```python
from build123d import *

# Parameters (mm, degrees)
SKETCH1_R           = 5
SKETCH1_R_2         = 6
SKETCH1_R_3         = 3
SKETCH1_R_4         = 4
BOSS_EXTRUDE1_DEPTH = 8


with BuildPart() as part:
    # Sketch1 → Boss-Extrude1 (new body)
    # profile 1 of 3: a face of its own
    with BuildSketch(Plane.XY):
        with BuildLine():
            Line((13.16300623, -179.16324922), (6, -179.16324922))
            ThreePointArc((6, -179.16324922), (4.585786438, -178.577462783), (4, -177.16324922))
            Line((4, -177.16324922), (4, -6.92820323))
            ThreePointArc((4, -6.92820323), (0, 8), (-4, -6.92820323))
            Line((-4, -6.92820323), (-4, -177.16324922))
            ThreePointArc((-4, -177.16324922), (-4.585786438, -178.577462783), (-6, -179.16324922))
            Line((-6, -179.16324922), (-12.83699377, -179.16324922))
            Line((-12.83699377, -179.16324922), (-12.83699377, -199.16324922))
            Line((-12.83699377, -199.16324922), (13.16300623, -199.16324922))
            Line((13.16300623, -199.16324922), (13.16300623, -179.16324922))
        make_face()
        Circle(SKETCH1_R, mode=Mode.SUBTRACT)
        with Locations((0.16300623, -189.16324922)):
            Circle(SKETCH1_R_2, mode=Mode.SUBTRACT)
        with BuildLine():
            ThreePointArc((-2, -175.16324922), (0, -177.16324922), (2, -175.16324922))
            Line((2, -175.16324922), (2, -11.176871049))
            ThreePointArc((2, -11.176871049), (0, -8.621835967), (-2, -11.176871049))
            Line((-2, -11.176871049), (-2, -175.16324922))
        make_face(mode=Mode.SUBTRACT)
    # profile 2 of 3: a face of its own
    with BuildSketch(Plane.XY):
        Circle(SKETCH1_R)
        Circle(SKETCH1_R_3, mode=Mode.SUBTRACT)
    # profile 3 of 3: a face of its own
    with BuildSketch(Plane.XY):
        with Locations((0.16300623, -189.16324922)):
            Circle(SKETCH1_R_2)
        with Locations((0.16300623, -189.16324922)):
            Circle(SKETCH1_R_4, mode=Mode.SUBTRACT)
    extrude(amount=BOSS_EXTRUDE1_DEPTH)


solid = part.part
```
Check sheet for the modelled part. Datum: model origin and axes. Units: mm. A direction names the side the tool comes from. Round coordinates to 2 decimals unless told otherwise and drop trailing zeros. Loops run counter-clockwise (first coordinate to the right, second up) from the corner with the lowest first, then second, coordinate; pieces in that order, holes last. Notation, with made-up numbers: (76.5, 24.5) - (91.5, 24.5) arc R19 cw to (91.5, 34.5) - close; hole circle Ø3 at (71, -37.75). An arc over 180 degrees is marked (long way). Write item = value, one per line. Start each with the question number.
Q1. Section check A-A (y = 0). Record the boundary of the cut face in (x, z).
Q2. Release check for a two-part mould opening along X. For faces 4 (the face through (2.31, -185.79, 3.94)), 5 (the face through (-9, -179.163, 4)), 6 (the face through (0, 8, 4)) record: pulls with the +X half, pulls with the -X half, needs draft (parallel to the pull), parting line crosses it, or undercut.
Q3. Thickness scan on L1, parallel to Y at x = 0, z = 4; L2, parallel to X at y = -33, z = 2; L3, parallel to Y at x = 12.25, z = 5.5. Record the ranges inside material, lowest first.
Q4. Section check C-C (y = -114.5). Record the boundary of the cut face in (x, z), plus the area to 3 significant figures.
Q5. Depth check by flat-ended pin: P1, Ø3, axis at x = 7.5, z = 5, coming from the +Y side; P2, Ø4, axis at y = -99, z = 4.5, coming from the -X side. Enter the tip coordinate at first touch or a pass-through.
Q6. Access from +Z, -Z, +X, -X, +Y, -Y to the whole of each face (thin tool, end or side, straight path). Record for faces 1 (the face through (4, -93, 4)), 2 (the face through (-0.044, -177.163, 3.944)), 3 (the face through (-4, -91, 4)).
Q7. Section check B-B (x = 0). Record the boundary of the cut face in (y, z).
Q8. Section check D-D (z = 2.5). Record the boundary of the cut face in (x, y), plus the area to 3 significant figures.
Derived:
q1.outline = (-8, 0) - (-3, 0) - (-3, 8) - (-8, 8) - close; (3, 0) - (8, 0) - (8, 8) - (3, 8) - close
q2.face_4 = undercut
q2.face_5 = needs draft
q2.face_6 = parting line crosses it
q3.L1 = -199.16 to -193.16, -185.17 to -177.16, -8.62 to -3, 3 to 8
q3.L2 = -4 to -2, 2 to 4
q3.L3 = -199.16 to -179.16
q4.outline = (-4, 0) - (-2, 0) - (-2, 8) - (-4, 8) - close; (2, 0) - (4, 0) - (4, 8) - (2, 8) - close
q4.area = 32.0 mm^2
q5.P1 = 5.29
q5.P2 = -4
q6.face_1 = +Z, -Z, +X
q6.face_2 = +Z, -Z
q6.face_3 = +Z, -Z, -X
q7.outline = (-199.16, 0) - (-193.16, 0) - (-193.16, 8) - (-199.16, 8) - close; (-185.17, 0) - (-177.16, 0) - (-177.16, 8) - (-185.17, 8) - close; (-8.62, 0) - (-3, 0) - (-3, 8) - (-8.62, 8) - close; (3, 0) - (8, 0) - (8, 8) - (3, 8) - close
q8.outline = (-12.84, -199.16) - (13.16, -199.16) - (13.16, -179.16) - (6, -179.16) arc R2 cw to (4, -177.16) - (4, -6.93) arc R8 ccw (long way) to (-4, -6.93) - (-4, -177.16) arc R2 cw to (-6, -179.16) - (-12.84, -179.16) - close; hole circle Ø8 at (0.16, -189.16); hole circle Ø6 at (0, 0); hole (-2, -175.16) arc R2 ccw to (2, -175.16) - (2, -11.18) arc R2.06 ccw (long way) to (-2, -11.18) - close
q8.area = 1,350 mm^2
